Check sheet for the modelled part. Datum: model origin and axes. Units: mm. A direction names the side the tool comes from. Coordinates: 2 decimals unless noted, no trailing zeros. Loops run counter-clockwise (first coordinate to the right, second up) from the corner with the lowest first, then second, coordinate; pieces in that order, holes last. Notation, with made-up numbers: (6, 47.25) - (35, 47.25) arc R16 ccw to (35, 68.25) - close; hole circle Ø10 at (48, 22.25). An arc over 180 degrees is marked (long way). Answer as a JSON object with one key per item and string values. Group by question number.
from build123d import *

# Parameters (mm, degrees)
M3X0_5_TAPPED_HOLE1_D     = 2.5
M3X0_5_TAPPED_HOLE1_DEPTH = 7.5
M3X0_5_TAPPED_HOLE1_TIP   = 0.751075774
CUT_EXTRUDE1_DEPTH        = 6
CIRPATTERN1_COUNT         = 4


with BuildPart() as part:
    # Sketch1 → Revolve1 (revolve)
    with BuildSketch(Plane.XY, mode=Mode.PRIVATE) as revolve1_sk:
        with BuildLine():
            Line((-2.5, 2), (-2.5, 0))
            Line((-2.5, 0), (-15, 0))
            ThreePointArc((-15, 0), (-23.778524933, 1.546556434), (-31.5, 6))
            Line((-31.5, 6), (-25.5, 6))
            Line((-25.5, 6), (-25.5, 16))
            Line((-25.5, 16), (-5, 16))
            Line((-5, 16), (-5, 4.5))
            Line((-5, 4.5), (-2.5, 2))
        make_face()
    revolve(revolve1_sk.sketch.rotate(Axis((0, 0, 0), (0, 1, 0)), 270), axis=Axis((0, 0, 0), (0, 1, 0)))

    # M3x0.5 Tapped Hole1
    with Locations(Plane(origin=(0, 0, 0), x_dir=(-1, 0, 0), z_dir=(0, -1, 0))):
        with Locations((12.5, 0), (-12.5, 0), (0, 12.5), (0, -12.5)):
            Hole(M3X0_5_TAPPED_HOLE1_D / 2, depth=M3X0_5_TAPPED_HOLE1_DEPTH)
            with Locations((0, 0, -(M3X0_5_TAPPED_HOLE1_DEPTH + M3X0_5_TAPPED_HOLE1_TIP / 2))):  # 118° drill point
                Cone(0, M3X0_5_TAPPED_HOLE1_D / 2, M3X0_5_TAPPED_HOLE1_TIP, mode=Mode.SUBTRACT)

    # Sketch4 → Cut-Extrude1 (cut)
    with BuildSketch(Plane.XZ):
        with BuildLine():
            Line((-5, -15.811388301), (-5, -22.79802623))
            ThreePointArc((-5, -22.79802623), (-6.034245075, -24.823257699), (-8.28125, -25.172820629))
            ThreePointArc((-8.28125, -25.172820629), (-18.738329701, -18.738329701), (-25.172820629, -8.28125))
            ThreePointArc((-25.172820629, -8.28125), (-24.823257699, -6.034245075), (-22.79802623, -5))
            Line((-22.79802623, -5), (-15.811388301, -5))
            ThreePointArc((-15.811388301, -5), (-14.475082091, -5.387114363), (-13.552618544, -6.428571429))
            ThreePointArc((-13.552618544, -6.428571429), (-10.606601718, -10.606601718), (-6.428571429, -13.552618544))
            ThreePointArc((-6.428571429, -13.552618544), (-5.387114363, -14.475082091), (-5, -15.811388301))
        make_face()
    cut_extrude1 = extrude(amount=-CUT_EXTRUDE1_DEPTH, mode=Mode.SUBTRACT)

    # CirPattern1: Cut-Extrude1 ×4 about axis
    cirpattern1_axis = Axis((0, 0, 0), (0, 1, 0))
    for i in range(1, CIRPATTERN1_COUNT):
        add(cut_extrude1.rotate(cirpattern1_axis, i * 360 / CIRPATTERN1_COUNT), mode=Mode.SUBTRACT)


solid = part.part
1. Sectioned sample at B-B on x = 18.5. State how many separate pieces and enclosed holes the cut face has, plus the area to 3 significant figures.
2. Release check for a two-part mould opening along X. For faces 4 (the face through (-19, 3, 5)), 5 (the face through (-26, 6, 2)) record: released by +X, released by -X, zero draft, split by the parting line, or undercut.
3. Sectioned sample at A-A on y = 14. Record the cut outline in (x, z), plus the area to 3 significant figures.
4. Gauge pin test, flat ends, axial feed: pin 1 (6 mm diameter, centred on x = 13, z = 17.5, fed in from -Y); pin 2 (6.5 mm diameter, centred on x = -19, y = 3.5, fed in from -Z); pin 3 (5 mm diameter, centred on x = 18.5, y = 2.5, fed in from +Z); pin 4 (3 mm diameter, centred on x = 0, z = 0, fed in from +Y). Record the tip position at first contact, or that the pin passes through.
5. Material ranges on line 1 (X direction, y = 13, z = 0); line 2 (X direction, y = 4.25, z = 12.5); line 3 (Z direction, x = -16.5, y = 5), recorded low to high.
6. Access from +Z, -Z, +X, -X, +Y, -Y to the whole of each face (thin tool, end or side, straight path). Record for faces 1 (the face through (24.84, 4.18, 6.06)), 2 (the face through (18.615, 4.336, 18.861)), 3 (the face through (3, 0, 0)).
Answers follow:
{
 "1": {"separate pieces": "3", "enclosed holes": "0", "area": "432 mm^2"},
 "2": {"face 4": "undercut", "face 5": "zero draft"},
 "3": {"outline": "circle Ø51 at (0, 0); hole circle Ø10 at (0, 0)", "area": "1,960 mm^2"},
 "4": {"pin 1": "stops at y = 6", "pin 2": "stops at z = -26.57", "pin 3": "stops at z = 24.29", "pin 4": "passes through"},
 "5": {"line 1": "x = -25.5 to -5, 5 to 25.5", "line 2": "x = -26.34 to -23.37, -8.29 to -1.25, 1.25 to 8.29, 23.37 to 26.34", "line 3": "z = -25.33 to -20.74, -5 to 5, 20.74 to 25.33"},
 "6": {"face 1": "-Y", "face 2": "+Y, -Y", "face 3": "+Z, -Z, +X, -X, -Y"}
}
